from build123d import *

# Parameters (mm, degrees)
F0_W         = 77.9
F0_H         = 158.2
F1_DEPTH     = 7.3
F2_R         = 5
F3_R         = 1.6899494937
F4_R         = 2.1727922061
F5_W         = 72.4303945899
F5_H         = 126.6588754952
F6_DEPTH     = 0.9
F7_R         = 5.0823894813
F8_DEPTH     = 0.9
F9_W         = 17.3039510846
F9_H         = 1.0814964771
F10_DEPTH    = 0.6
F11_R        = 0.8966339166
F12_DEPTH    = 0.8
F13_W        = 17.3039520159
F13_H        = 4.6321238935
F14_DEPTH    = 1.7
F15_R        = 0.7242640687
F16_R        = 1.0910584654
F17_DEPTH    = 1.2
F18_R        = 1.1204591048
F18_R_2      = 0.2597799208
F19_DEPTH    = 0.5
F20_R        = 0.5652467708
F21_DEPTH    = 1.3
F22_R        = 1.5140930758
F23_DEPTH    = 0.6
F24_W        = 10.0857308134
F24_H        = 1.8002798315
F25_DEPTH    = 8.7
F26_W        = 7.992297411
F26_H        = 1.5090261586
F27_DEPTH    = 0.5
F28_T1_DEPTH = 5.0389206483
F28_T3_DEPTH = 11.5221919007
F29_R        = 1.0914541248
F30_DEPTH    = 0.9
F31_R        = 1.1331057204
F32_DEPTH    = 0.8
F33_W        = 73.5544155877
F33_H        = 1.0814964771
F34_DEPTH    = 0.4


# Not quite as in the source:
# - a fillet or chamfer that OpenCascade refuses, or shapes differently, is made with other operations: its cross-section is extruded or revolved along the edge and cut away or added


with BuildPart() as f1:
    # F0 (on Top) → F1 (new body)
    with BuildSketch(Plane.XY):
        with Locations((-9.3765874773, -13.58352229)):
            Rectangle(F0_W, F0_H)
    extrude(amount=F1_DEPTH)

    # F2
    f2_edges = [f1.edges().sort_by_distance(p)[0] for p in [
        (-48.326587, -92.683522, 3.65),
        (29.573413, -92.683522, 3.65),
        (29.573413, 65.516478, 3.65),
        (-48.326587, 65.516478, 3.65),
    ]]
    fillet(f2_edges, radius=F2_R)

    # F3
    f3_edges = [f1.edges().sort_by_distance(p)[0] for p in [
        (-48.326587, -13.583522, 7.3),
        (-9.376587, 65.516478, 7.3),
        (28.108946, 64.052012, 7.3),
        (-46.862121, 64.052012, 7.3),
        (29.573413, -13.583522, 7.3),
        (28.108946, -91.219056, 7.3),
        (-46.862121, -91.219056, 7.3),
        (-9.376587, -92.683522, 7.3),
    ]]
    fillet(f3_edges, radius=F3_R)

    # F4
    f4_edges = [f1.edges().sort_by_distance(p)[0] for p in [
        (-48.326587, -13.583522, 0),
        (-9.376587, 65.516478, 0),
        (28.108946, 64.052012, 0),
        (-46.862121, 64.052012, 0),
        (29.573413, -13.583522, 0),
        (28.108946, -91.219056, 0),
        (-46.862121, -91.219056, 0),
        (-9.376587, -92.683522, 0),
    ]]
    fillet(f4_edges, radius=F4_R)

    # F5 (on face) → F6 (cut)
    with BuildSketch(Plane.XY.offset(7.3)):
        with Locations((-9.5828361809, -11.9932051748)):
            Rectangle(F5_W, F5_H)
    extrude(amount=-F6_DEPTH, mode=Mode.SUBTRACT)

    # F7 (on face) → F8 (cut)
    with BuildSketch(Plane.XY.offset(7.3)):
        with Locations((-9.5828361809, -83.671361208)):
            Circle(F7_R)
    extrude(amount=-F8_DEPTH, mode=Mode.SUBTRACT)

    # F9 (on face) → F10 (cut)
    with BuildSketch(Plane.XY.offset(7.3)):
        with Locations((-8.6519755423, 57.6703026891)):
            Rectangle(F9_W, F9_H)
    extrude(amount=-F10_DEPTH, mode=Mode.SUBTRACT)

    # F11 (on face) → F12 (cut)
    with BuildSketch(Plane.XY.offset(7.3)):
        with Locations((-22.4402733147, 57.7334612608)):
            Circle(F11_R)
    extrude(amount=-F12_DEPTH, mode=Mode.SUBTRACT)

    # F13 (on face) → F14 (join)
    with BuildSketch(Plane(origin=(0, 0, 0), x_dir=(1, 0, 0), z_dir=(0, 0, -1))):
        with Locations((11.9729838334, -58.2004157633)):
            Rectangle(F13_W, F13_H)
    extrude(amount=F14_DEPTH)

    # F15
    f15_edges = [f1.edges().sort_by_distance(p)[0] for p in [
        (11.972984, 60.516478, -1.7),
        (11.972984, 55.884354, -1.7),
        (20.62496, 58.200416, -1.7),
        (3.321008, 58.200416, -1.7),
    ]]
    fillet(f15_edges, radius=F15_R)

    # F16 (on face) → F17 (cut)
    with BuildSketch(Plane(origin=(0, 0, -1.7), x_dir=(1, 0, 0), z_dir=(0, 0, -1))):
        with Locations((17.652342096, -58.0027028918)):
            Circle(F16_R)
    extrude(amount=-F17_DEPTH, mode=Mode.SUBTRACT)

    # F18 (on face) → F19 (cut)
    with BuildSketch(Plane(origin=(0, 0, -1.7), x_dir=(1, 0, 0), z_dir=(0, 0, -1))):
        with Locations((13.1328506395, -57.9593703151)):
            Circle(F18_R)
        with Locations((13.1328506395, -57.9593703151)):
            Circle(F18_R_2, mode=Mode.SUBTRACT)
    extrude(amount=-F19_DEPTH, mode=Mode.SUBTRACT)

    # F20 (on face) → F21 (cut)
    with BuildSketch(Plane(origin=(0, 0, 0), x_dir=(1, 0, 0), z_dir=(0, 0, -1))):
        with Locations((0, -57.881783694)):
            Circle(F20_R)
    extrude(amount=-F21_DEPTH, mode=Mode.SUBTRACT)

    # F22 (on face) → F23 (cut)
    with BuildSketch(Plane(origin=(0, 0, 0), x_dir=(1, 0, 0), z_dir=(0, 0, -1))):
        with Locations((-3.8621318527, -57.8266605735)):
            Circle(F22_R)
    extrude(amount=-F23_DEPTH, mode=Mode.SUBTRACT)

    # F24 (on face) → F25 (cut)
    with BuildSketch(Plane.XZ.offset(92.68352229)):
        with Locations((-9.6801561303, 3.9914349327)):
            Rectangle(F24_W, F24_H)
    extrude(amount=-F25_DEPTH, mode=Mode.SUBTRACT)

    # F26 (on face) → F27 (join)
    with BuildSketch(Plane.YZ.offset(29.5734125227)):
        with Locations((42.0706942677, 3.8539019879)):
            Rectangle(F26_W, F26_H)
    extrude(amount=F27_DEPTH)

    # F28: fillet of radius 0.7484062043 on 4 edges, made by hand

    # F28_s2 → F28_t1 (cut)
    with BuildSketch(Plane.XY.offset(1.3344416637)):
        with BuildLine():
            ThreePointArc((29.5734125227, 46.0668429732), (29.9357520066, 45.7934164433), (30.0734125227, 45.3608640753))
            Line((30.0734125227, 45.3608640753), (30.0734125227, 46.0668429732))
            Line((30.0734125227, 46.0668429732), (29.5734125227, 46.0668429732))
        make_face()
        with BuildLine():
            ThreePointArc((29.5734125227, 38.0745455623), (29.9357520066, 38.3479720922), (30.0734125227, 38.7805244602))
            Line((30.0734125227, 38.7805244602), (30.0734125227, 38.0745455623))
            Line((30.0734125227, 38.0745455623), (29.5734125227, 38.0745455623))
        make_face()
    extrude(amount=F28_T1_DEPTH, mode=Mode.SUBTRACT)

    # F28_s4 → F28_t3 (cut)
    with BuildSketch(Plane.XZ.offset(-47.8317902181)):
        with BuildLine():
            ThreePointArc((29.5734125227, 4.6084150672), (29.9357520066, 4.3349885373), (30.0734125227, 3.9024361693))
            Line((30.0734125227, 3.9024361693), (30.0734125227, 4.6084150672))
            Line((30.0734125227, 4.6084150672), (29.5734125227, 4.6084150672))
        make_face()
        with BuildLine():
            ThreePointArc((29.5734125227, 3.0993889086), (29.9357520066, 3.3728154385), (30.0734125227, 3.8053678065))
            Line((30.0734125227, 3.8053678065), (30.0734125227, 3.0993889086))
            Line((30.0734125227, 3.0993889086), (29.5734125227, 3.0993889086))
        make_face()
    extrude(amount=F28_T3_DEPTH, mode=Mode.SUBTRACT)

    # F29 (on face) → F30 (join)
    with BuildSketch(Plane(origin=(-48.3265874773, 0, 0), x_dir=(0, -1, 0), z_dir=(-1, 0, 0))):
        with Locations((-41.7392961681, 4.070978146)):
            Circle(F29_R)
    extrude(amount=F30_DEPTH)

    # F31 (on face) → F32 (join)
    with BuildSketch(Plane(origin=(-48.3265874773, 0, 0), x_dir=(0, -1, 0), z_dir=(-1, 0, 0))):
        with Locations((-36.7904044688, 4.1209622286)):
            Circle(F31_R)
    extrude(amount=F32_DEPTH)

    # F33 (on face) → F34 (cut)
    with BuildSketch(Plane(origin=(0, 0, 0), x_dir=(1, 0, 0), z_dir=(0, 0, -1))):
        with Locations((-9.3765874773, 75.3538236022)):
            Rectangle(F33_W, F33_H)
    extrude(amount=-F34_DEPTH, mode=Mode.SUBTRACT)


solid = f1.part
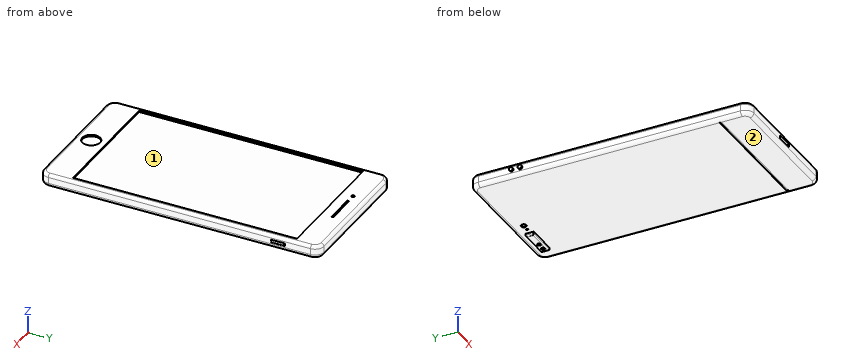
Can you work these out from the model? Positions are in its coordinate system, mm. Face numbers are marked on the shaded views. Round coordinates to 2 decimals unless told otherwise and drop trailing zeros. Write each loop counter-clockwise with the first axis right and the second up, starting at its lowest first coordinate (ties: lowest second). Pieces come first, ordered by that corner, then holes. Notation, with made-up numbers: M -10,-24.75 L 29,-24.75 A29 ccw 29,-0.75 Z; hole C -9.5,34.25 d7. An arc over 180 degrees is marked long. Use CSV: the item, a comma, the result in double quotes.
(1) Imagine slicing it at B-B (x = 7.5). Write out the boundary of the cut face in (y, z), plus the area to 3 significant figures.
Check values:
outline,"M -92.68,2.17 A2.17 ccw -90.51,0 L -75.89,0 L -75.89,0.4 L -74.81,0.4 L -74.81,0 L 55.88,0 L 55.88,-0.98 A0.72 ccw 56.61,-1.7 L 59.79,-1.7 A0.72 ccw 60.52,-0.98 L 60.52,0 L 63.34,0 A2.17 ccw 65.52,2.17 L 65.52,5.61 A1.69 ccw 63.83,7.3 L 51.34,7.3 L 51.34,6.4 L -75.32,6.4 L -75.32,7.3 L -90.99,7.3 A1.69 ccw -92.68,5.61 Z"
area,"1,040 mm^2"
(2) I'm going to push flat-ended pins straight in: pin 1 (0.8 mm diameter, centred on y = 57.5, z = -0.5, fed in from -X); pin 2 (0.9 mm diameter, centred on x = -20, y = -75, fed in from -Z); pin 3 (0.5 mm diameter, centred on x = -9, z = 4, fed in from -Y). Where does each tip first touch, or does it pass through?
Check values:
pin 1,"x = 3.32"
pin 2,"z = 0"
pin 3,"y = -83.98"
(3) Imagine slicing it at A-A (y = -51.5). Write out the boundary of the cut face in (x, z), plus the area to 3 significant figures.
Check values:
outline,"M -48.33,2.17 A2.17 ccw -46.15,0 L 27.4,0 A2.17 ccw 29.57,2.17 L 29.57,5.61 A1.69 ccw 27.88,7.3 L 26.63,7.3 L 26.63,6.4 L -45.8,6.4 L -45.8,7.3 L -46.64,7.3 A1.69 ccw -48.33,5.61 Z"
area,"500 mm^2"
(4) I need wall thicknesses on line 1 along Z through (x, y) = (-14, -84.5); line 2 along X through (y, z) = (-41, 4); line 3 along Z through (x, y) = (-43.5, -51.5). Which ranges of each line are inside material? Lowest first, please.
Check values:
line 1,"0 to 3.09, 4.89 to 6.4"
line 2,"-48.33 to 29.57"
line 3,"0 to 6.4"
(5) We'd pull the mould along X, two halves only. Please class the marked faces 1 and 2: +X half, -X half, draft (parallel to the pull), parting line (faces both ways), or undercut.
Check values:
face 1,"undercut"
face 2,"draft"
